from build123d import *

# Parameters (mm, degrees)
CHAMFER_1_SIZE      = 0.5
CUT_EXTRUDE_1_DEPTH = 2.5


with BuildPart() as part:
    # 草图1 → 旋转1 (revolve)
    with BuildSketch(Plane(origin=(0, 0, 0), x_dir=(0, 0, -1), z_dir=(1, 0, 0))):
        Polygon((-6, 0), (-6, 4), (-5.4, 4), (-3.4, 2), (6, 2), (6, 0), align=None)
    revolve(axis=Axis((0, 0, -6), (0, 0, 1)))

    # 倒角1
    chamfer_1_edges = [part.edges().sort_by_distance(p)[0] for p in [
        (0, -2, -6),
    ]]
    chamfer(chamfer_1_edges, length=CHAMFER_1_SIZE)

    # 草图2 → 切除-拉伸1 (cut)
    with BuildSketch(Plane.XY.offset(6)):
        Polygon((0, 1.443375673), (-1.25, 0.721687836), (-1.25, -0.721687836), (0, -1.443375673), (1.25, -0.721687836), (1.25, 0.721687836), align=None)
    extrude(amount=-CUT_EXTRUDE_1_DEPTH, mode=Mode.SUBTRACT)


solid = part.part
Geometry check sheet. Reference: the model listing, model coordinates, mm. A direction names the side the tool comes from. Round coordinates to 2 decimals unless told otherwise and drop trailing zeros. Order: outer loops, then holes, each group sorted by start corner. A loop starts at its lowest first (then second) coordinate and runs counter-clockwise, first axis right, second up. Notation, with made-up numbers: (61.25, 57.5) -> (94.25, 57.5) arc R25 cw to (94.25, 79.5) -> close; hole circle Ø11 at (22.25, -15.5). An arc over 180 degrees is marked (long way). Use one line per item in the form item = value.
1. Mould release check, pull along Y, two halves, no side actions. Record for faces 3 (the face through (2, 0, -1)), 4 (the face through (0.63, 1.08, 4.77)), 5 (the face through (0, -2, 6)): pulls with the +Y half, pulls with the -Y half, needs draft (parallel to the pull), parting line crosses it, or undercut.
Working result:
face_3 = parting line crosses it
face_4 = undercut
face_5 = needs draft
2. Set-up check for faces 1 (the face through (0, 0, -6)), 2 (the face through (0.616, -1.088, 4.768)): record each of +Z, -Z, +X, -X, +Y, -Y from which the full face is reachable in a straight line by a thin tool's end or side.
Working result:
face_1 = -Z, +X, -X, +Y, -Y
face_2 = +Z
3. Go/stop test with flat-tipped pins: pin 1 (1.5 mm diameter, centred on x = 3, y = 3, fed in from -Z); pin 2 (0.7 mm diameter, centred on y = 0, z = 4.5, fed in from -X); pin 3 (2 mm diameter, centred on x = -2.5, z = -5, fed in from +Y). Record where each tip stops, or that it passes through.
Working result:
pin_1 = 4.89
pin_2 = -3.45
pin_3 = 1.32
4. Cross-section at B-B, the plane z = 3. Enter the section's corners in (x, y), plus the area to 3 significant figures.
Working result:
outline = circle Ø4 at (0, 0)
area = 12.6 mm^2
5. Cross-section at A-A, the plane y = 0. Enter the section's corners in (x, z).
Working result:
outline = (-4, 5.4) -> (-2, 3.4) -> (-2, -5.5) -> (-1.5, -6) -> (1.5, -6) -> (2, -5.5) -> (2, 3.4) -> (4, 5.4) -> (4, 6) -> (1.25, 6) -> (1.25, 3.5) -> (-1.25, 3.5) -> (-1.25, 6) -> (-4, 6) -> close
6. Scan lines: line 1 along Z through (x, y) = (-0.5, 0.5); line 2 along Y through (x, z) = (0, 2.5); line 3 along Z through (x, y) = (-1.25, 3). Record each from-to range of solid material in increasing order. Write a range as from..to.
Working result:
line_1 = -6..3.5
line_2 = -2..2
line_3 = 4.65..6
